Source: three-view drawing plus pictorial views. Frame: mm from the lowest corner of the part. A direction names the side the tool comes from. Give positions to 0.01 mm unless a question says otherwise; leave off trailing zeros. Loops run counter-clockwise (first coordinate to the right, second up) from the corner with the lowest first, then second, coordinate; pieces in that order, holes last. Notation, with made-up numbers: (65.25, 85.25) - (123.25, 85.25) arc R21 cw to (123.25, 119.25) - close; hole circle Ø6 at (18, 30). An arc over 180 degrees is marked (long way). Write each question's results on one line, items separated by ' | '. Start each with the question number.
(1) Pull-direction query (X, two-part tool) for the marked faces 1, 2 and 3; classes: pulls with the +X half, pulls with the -X half, needs draft (parallel to the pull), parting line crosses it, or undercut.
(2) Cut plane B-B on x = 2.25. Return the cut outline in (y, z).
(3) Reachability of the marked faces 4, 5 and 6 from +Z, -Z, +X, -X, +Y, -Y: full face, straight path, thin tool, end or side. Return the list, or none.
(4) Cut plane C-C on z = 11.5. Return the cut outline in (x, y).
(5) Cut plane D-D on z = 4.75. Return the cut outline in (x, y).
(6) Contact query for a flat-ended pin moving along its axis: pin 1 (6 mm diameter, centred on x = 6.5, z = 10, fed in from -Y). Output: stop coordinate, or through.
(7) Material intervals for line 1 along X through (y, z) = (2.5, 19); line 2 along Z through (x, y) = (1.5, 10); line 3 along Y through (x, z) = (10.5, 14.25), sorted ascending. Write a range as [from, to].
(8) Cut plane A-A on y = 7.5. Return the cut outline in (x, z), then the cut area to 3 significant figures.
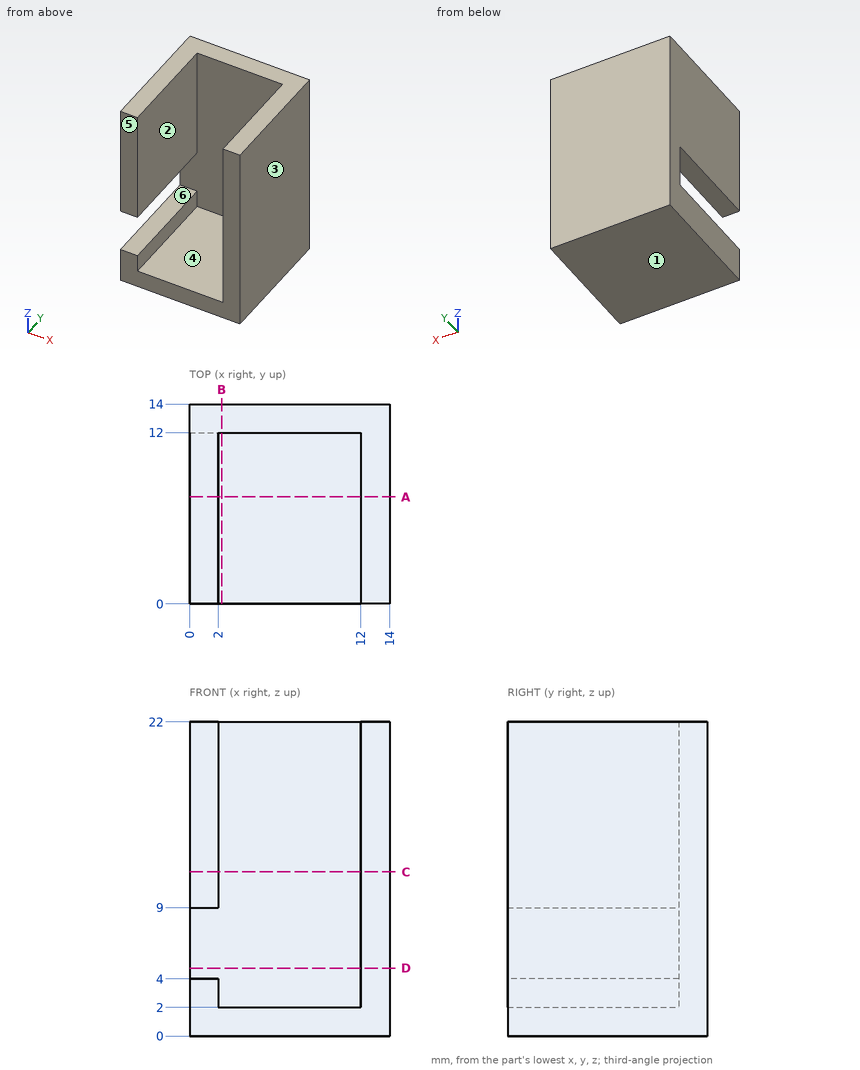
Ans:
1) face 1: needs draft | face 2: undercut | face 3: pulls with the +X half
2) outline: (0, 0) - (14, 0) - (14, 22) - (12, 22) - (12, 2) - (0, 2) - close
3) face 4: +Z, -Y | face 5: +Z, -Z, +X, -X, -Y | face 6: -X, -Y
4) outline: (0, 0) - (2, 0) - (2, 12) - (12, 12) - (12, 0) - (14, 0) - (14, 14) - (0, 14) - close
5) outline: (0, 12) - (12, 12) - (12, 0) - (14, 0) - (14, 14) - (0, 14) - close
6) pin 1: y = 12
7) line 1: [0, 2], [12, 14] | line 2: [0, 4], [9, 22] | line 3: [12, 14]
8) outline: (0, 0) - (14, 0) - (14, 22) - (12, 22) - (12, 2) - (2, 2) - (2, 4) - (0, 4) - close; (0, 9) - (2, 9) - (2, 22) - (0, 22) - close | area: 98.0 mm^2
